Build history of the part. All positions in model axes, mm. A direction names the side the tool comes from. Round coordinates to 2 decimals unless told otherwise and drop trailing zeros. Order: outer loops, then holes, each group sorted by start corner. A loop starts at its lowest first (then second) coordinate and runs counter-clockwise, first axis right, second up. Notation, with made-up numbers: M 59.25,75.5 L 96.25,75.5 A18 cw 96.25,98.5 Z; hole C 15.5,-32 d6. An arc over 180 degrees is marked long. One line per item, written item: value. Start each with the question number.
Item 1: Pin check, flat tips, straight feed: pin 1 (0.9 mm diameter, centred on y = 6.5, z = 3, fed in from -X); pin 2 (3 mm diameter, centred on x = 4.5, z = 1.5, fed in from +Y); pin 3 (1.5 mm diameter, centred on y = 6.5, z = 4, fed in from +X). Stop position of each tip, or through.
Item 2: Two-plate mould, pull along Y, no slides. Class faces 1 (the flat face through (0, 0, 2)), 2 (the flat face through (0, -9, 1)), 3 (the flat face through (-7.5, 0, 1)): +Y half, -Y half, draft (parallel to the pull), parting line (faces both ways), or undercut.
Item 3: Tool access for faces 4 (the flat face through (2, 8, 3)), 5 (the flat face through (0, -11, 2)), 6 (the flat face through (0, -6.5, 3)): list every direction of +Z, -Z, +X, -X, +Y, -Y with a clear straight run to the whole face (end or side of a thin tool).
Item 4: Band-saw the part on B-B, the plane x = 5.5. Write the cut outline in (y, z), then the cut area to 3 significant figures.
Item 5: Band-saw the part on D-D, the plane x = -3. Write the cut outline in (y, z).
Item 6: Probe L1, parallel to Y at x = -5.5, z = 1.4; L2, parallel to Y at x = 1, z = 3.45; L3, parallel to Z at x = -2, y = -4. List the from-to ranges inside material, lowest first.
Item 7: Band-saw the part on C-C, the plane y = 3. Write the cut outline in (x, z).
Item 8: Band-saw the part on A-A, the plane z = 3.25. Write the cut outline in (x, y), then the cut area to 3 significant figures.
```python
from build123d import *

# Parameters (mm, degrees)
CROQUIS1_W              = 15
CROQUIS1_H              = 18
SALIENTE_EXTRUIR1_DEPTH = 2
CROQUIS2_R              = 1.5
CORTAR_EXTRUIR1_DEPTH   = 12.884864324
CROQUIS3_W              = 4
CROQUIS3_H              = 12
SALIENTE_EXTRUIR2_DEPTH = 3
CROQUIS4_W              = 8
CROQUIS4_H              = 7
SALIENTE_EXTRUIR3_DEPTH = 3


with BuildPart() as part:
    # Croquis1 → Saliente-Extruir1 (new body)
    with BuildSketch(Plane.XY):
        Rectangle(CROQUIS1_W, CROQUIS1_H)
    extrude(amount=SALIENTE_EXTRUIR1_DEPTH)

    # Croquis2 → Cortar-Extruir1 (cut, through all)
    with BuildSketch(Plane.XY.offset(2)):
        with Locations((-5.5, 7)):
            Circle(CROQUIS2_R)
        with Locations((5.5, 7)):
            Circle(CROQUIS2_R)
    extrude(amount=-CORTAR_EXTRUIR1_DEPTH, mode=Mode.SUBTRACT)

    # Croquis3 → Saliente-Extruir2 (add)
    with BuildSketch(Plane.XY.offset(2)):
        with Locations((0, 8)):
            Rectangle(CROQUIS3_W, CROQUIS3_H)
    extrude(amount=SALIENTE_EXTRUIR2_DEPTH)

    # Croquis4 → Saliente-Extruir3 (add)
    with BuildSketch(Plane.XY.offset(2)):
        with Locations((0, -10)):
            Rectangle(CROQUIS4_W, CROQUIS4_H)
    extrude(amount=SALIENTE_EXTRUIR3_DEPTH)


solid = part.part
```
Output:
1. pin 1: stops at x = -2
1. pin 2: stops at y = 9
1. pin 3: stops at x = 2
2. face 1: undercut
2. face 2: -Y half
2. face 3: draft
3. face 4: +Z, +X, +Y
3. face 5: -Z, +X, -X, -Y
3. face 6: +Z, +X, -X
4. outline: M -9,0 L 5.5,0 L 5.5,2 L -9,2 Z; M 8.5,0 L 9,0 L 9,2 L 8.5,2 Z
4. area: 30.0 mm²
5. outline: M -13.5,2 L -9,2 L -9,0 L 9,0 L 9,2 L -6.5,2 L -6.5,5 L -13.5,5 Z
6. L1: y = -9 to 5.5, 8.5 to 9
6. L2: y = -13.5 to -6.5, 2 to 14
6. L3: z = 0 to 2
7. outline: M -7.5,0 L 7.5,0 L 7.5,2 L 2,2 L 2,5 L -2,5 L -2,2 L -7.5,2 Z
8. outline: M -4,-13.5 L 4,-13.5 L 4,-6.5 L -4,-6.5 Z; M -2,2 L 2,2 L 2,14 L -2,14 Z
8. area: 104 mm²
